Part model, mm, in its own coordinate system. Face numbers are marked on the shaded views. A direction names the side the tool comes from. Round coordinates to 2 decimals unless told otherwise and drop trailing zeros. Order: outer loops, then holes, each group sorted by start corner. A loop starts at its lowest first (then second) coordinate and runs counter-clockwise, first axis right, second up. Notation, with made-up numbers: (32.5, -13.5) - (58.5, -13.5) arc R9 ccw to (58.5, 1.5) - close; hole circle Ø1 at (58.25, 80.5). An arc over 180 degrees is marked (long way). Return JSON: item names as keys, results as strings. Group by question number.
Item 1: Probe probe 1 along X at (y, z) = (96.9, 30); probe 2 along Z at (x, y) = (324, 96.65); probe 3 along Y at (x, z) = (287.5, -9). List the from-to ranges inside material, lowest first.
Item 2: Tool access for the marked faces 4 and 5: list every direction of +Z, -Z, +X, -X, +Y, -Y with a clear straight run to the whole face (end or side of a thin tool).
Item 3: Saw through at D-D on y = 105. List the corners of the cut face in (x, z).
Item 4: Saw through at B-B on x = 324. List the corners of the cut face in (y, z).
Item 5: Drop flat-ended pins along their axis: pin 1 (1.5 mm diameter, centred on x = 308.5, y = 106.5, fed in from -Z); pin 2 (2.5 mm diameter, centred on x = 301, y = 105.5, fed in from +Z); pin 3 (4 mm diameter, centred on x = 324, z = -30, fed in from +Y). Give the stop position or say it passes through.
Item 6: Saw through at C-C on z = 0. List the corners of the cut face in (x, y), and give its area (3 significant figures).
Item 7: Two-plate mould, pull along X, no slides. Class the marked faces 1, 2 and 3: released by +X, released by -X, zero draft, split by the parting line, or undercut.
Item 8: Saw through at A-A on z = 30. List the corners of the cut face in (x, y), and give its area (3 significant figures).
```python
from build123d import *

# Parameters (mm, degrees)
CROQUIS1_W                                           = 45
CROQUIS1_H                                           = 66
SALIENTE_EXTRUIR1_DEPTH                              = 3
REDONDEO1_R                                          = 2
CROQUIS2_W                                           = 25
CROQUIS2_H                                           = 46
SALIENTE_EXTRUIR2_DEPTH                              = 10
REDONDEO2_R                                          = 5
REDONDEO3_R                                          = 5
AVELLANADO_PARA_TORNILLO_CON_CABEZA_OVAL_D           = 6.7564
AVELLANADO_PARA_TORNILLO_CON_CABEZA_OVAL_CSINK_D     = 12.8778
AVELLANADO_PARA_TORNILLO_CON_CABEZA_OVAL_CSINK_ANGLE = 82
TALADRO_DE_MARGEN_PARA_M31_D                         = 3.4


with BuildPart() as part:
    # Croquis1 → Saliente-Extruir1 (new body)
    with BuildSketch(Plane(origin=(0, 95.1, 0), x_dir=(1, 0, 0), z_dir=(0, 1, 0))):
        with Locations((305.171572875, 0)):
            Rectangle(CROQUIS1_W, CROQUIS1_H)
        with BuildLine():
            ThreePointArc((323.15, 30), (324, 29.15), (324.85, 30))
            ThreePointArc((324.85, 30), (324, 30.85), (323.15, 30))
        make_face(mode=Mode.SUBTRACT)
        with BuildLine():
            ThreePointArc((285.65, 30), (286.5, 29.15), (287.35, 30))
            ThreePointArc((287.35, 30), (286.5, 30.85), (285.65, 30))
        make_face(mode=Mode.SUBTRACT)
        with BuildLine():
            ThreePointArc((285.65, -30), (286.5, -30.85), (287.35, -30))
            ThreePointArc((287.35, -30), (286.5, -29.15), (285.65, -30))
        make_face(mode=Mode.SUBTRACT)
        with BuildLine():
            ThreePointArc((323.15, -30), (324, -30.85), (324.85, -30))
            ThreePointArc((324.85, -30), (324, -29.15), (323.15, -30))
        make_face(mode=Mode.SUBTRACT)
    extrude(amount=SALIENTE_EXTRUIR1_DEPTH)

    # Redondeo1
    redondeo1_edges = [part.edges().sort_by_distance(p)[0] for p in [
        (282.671572875, 96.6, -33),
        (327.671572875, 96.6, -33),
        (327.671572875, 96.6, 33),
        (282.671572875, 96.6, 33),
    ]]
    fillet(redondeo1_edges, radius=REDONDEO1_R)

    # Croquis2 → Saliente-Extruir2 (add)
    with BuildSketch(Plane(origin=(0, 98.1, 0), x_dir=(1, 0, 0), z_dir=(0, 1, 0))):
        with Locations((305.171572875, 0)):
            Rectangle(CROQUIS2_W, CROQUIS2_H)
    extrude(amount=SALIENTE_EXTRUIR2_DEPTH)

    # Redondeo2
    redondeo2_edges = [part.edges().sort_by_distance(p)[0] for p in [
        (305.171572875, 98.1, -23),
        (305.171572875, 98.1, 23),
    ]]
    fillet(redondeo2_edges, radius=REDONDEO2_R)

    # Redondeo3
    redondeo3_edges = [part.edges().sort_by_distance(p)[0] for p in [
        (292.671572875, 98.1, 0),
        (317.671572875, 98.1, 0),
    ]]
    fillet(redondeo3_edges, radius=REDONDEO3_R)

    # Avellanado para tornillo con cabeza ovalada de 1/41 (through all)
    with Locations(Plane(origin=(0, 95.1, 0), x_dir=(-1, 0, 0), z_dir=(0, -1, 0))):
        with Locations((-305.171572875, 0)):
            CounterSinkHole(AVELLANADO_PARA_TORNILLO_CON_CABEZA_OVAL_D / 2, AVELLANADO_PARA_TORNILLO_CON_CABEZA_OVAL_CSINK_D / 2, counter_sink_angle=AVELLANADO_PARA_TORNILLO_CON_CABEZA_OVAL_CSINK_ANGLE)

    # Taladro de margen para M31 (through all)
    with Locations(Plane(origin=(0, 98.1, 0), x_dir=(1, 0, 0), z_dir=(0, 1, 0))):
        with Locations((324, -30), (286.5, -30), (324, 30), (286.5, 30)):
            Hole(TALADRO_DE_MARGEN_PARA_M31_D / 2)


solid = part.part
```
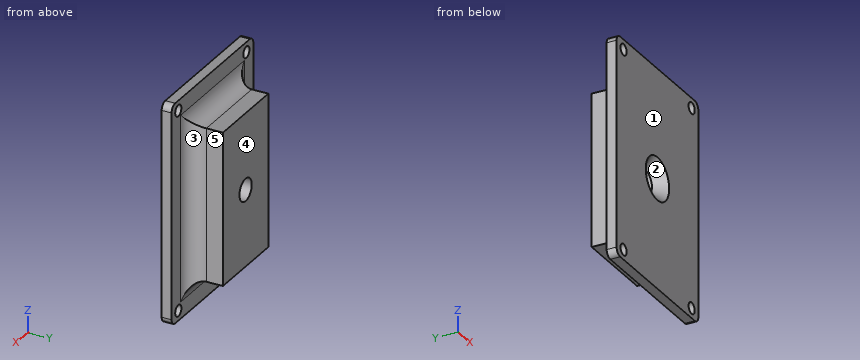
Filled in:
{
 "1": {"probe 1": "x = 282.67 to 284.8, 288.2 to 322.3, 325.7 to 327.67", "probe 2": "z = -33 to -31.7, -28.3 to 28.3, 31.7 to 33", "probe 3": "y = 95.1 to 98.1"},
 "2": {"face 4": "+Z, -Z, +X, -X, +Y", "face 5": "+Z, -Z, +X, +Y"},
 "3": {"outline": "(292.67, -23) - (317.67, -23) - (317.67, 23) - (292.67, 23) - close; hole circle Ø6.76 at (305.17, 0)"},
 "4": {"outline": "(95.1, -33) - (98.1, -33) - (98.1, -31.7) - (95.1, -31.7) - close; (95.1, -28.3) - (98.1, -28.3) - (98.1, 28.3) - (95.1, 28.3) - close; (95.1, 31.7) - (98.1, 31.7) - (98.1, 33) - (95.1, 33) - close"},
 "5": {"pin 1": "stops at z = -23", "pin 2": "stops at z = 23", "pin 3": "stops at y = 98.1"},
 "6": {"outline": "(282.67, 95.1) - (298.73, 95.1) - (301.79, 98.62) - (301.79, 108.1) - (292.67, 108.1) - (292.67, 103.1) arc R5 cw to (287.67, 98.1) - (282.67, 98.1) - close; (308.55, 98.62) - (311.61, 95.1) - (327.67, 95.1) - (327.67, 98.1) - (322.67, 98.1) arc R5 cw to (317.67, 103.1) - (317.67, 108.1) - (308.55, 108.1) - close", "area": "297 mm^2"},
 "7": {"face 1": "zero draft", "face 2": "undercut", "face 3": "released by +X"},
 "8": {"outline": "(282.67, 95.1) - (284.8, 95.1) - (284.8, 98.1) - (282.67, 98.1) - close; (288.2, 95.1) - (322.3, 95.1) - (322.3, 98.1) - (288.2, 98.1) - close; (325.7, 95.1) - (327.67, 95.1) - (327.67, 98.1) - (325.7, 98.1) - close", "area": "115 mm^2"}
}
